Here's how the part is built. I have some questions about the finished solid (model axes, mm). Give positions to 0.01 mm unless a question says otherwise; leave off trailing zeros. Order: outer loops, then holes, each group sorted by start corner. A loop starts at its lowest first (then second) coordinate and runs counter-clockwise, first axis right, second up.
from build123d import *

# Parameters (mm, degrees)
PAD007_DEPTH    = 12
SKETCH017_R     = 4
POCKET003_DEPTH = 12.001
SKETCH042_R     = 4
HOLE009_DEPTH   = 610.001


with BuildPart() as side_left_bottom_part:
    # Sketch016 → Pad007 (new body)
    with BuildSketch(Plane.YZ):
        with BuildLine():
            ThreePointArc((-597.560459, -4876.606763), (-519.72621, -4994.682239), (-401.650734, -4916.84799))
            ThreePointArc((-401.650734, -4916.84799), (-253.112342, -4128.51152), (-130.4314, -3335.739529))
            Line((-195.221935, -3317.531256), (-130.4314, -3335.739529))
            ThreePointArc((-199.003331, -3309.149426), (-199.067813, -3314.222405), (-195.221935, -3317.531256))
            Line((-175.537372, -3260.47474), (-199.003331, -3309.149426))
            ThreePointArc((-175.537372, -3260.47474), (-175.47289, -3255.401761), (-179.318768, -3252.09291))
            Line((-244.109303, -3233.884637), (-179.318768, -3252.09291))
            ThreePointArc((-244.109303, -3233.884637), (-249.326998, -3234.856662), (-251.732171, -3239.58787))
            Line((-252.389603, -3293.61975), (-251.732171, -3239.58787))
            ThreePointArc((-260.01247, -3299.322983), (-254.794775, -3298.350957), (-252.389603, -3293.61975))
            Line((-324.803005, -3281.114709), (-260.01247, -3299.322983))
            ThreePointArc((-597.560459, -4876.606763), (-447.909647, -4081.129666), (-324.803005, -3281.114709))
        make_face()
    extrude(amount=PAD007_DEPTH)

    # Sketch017 → Pocket003 (cut, through all)
    with BuildSketch(Plane.YZ):
        with Locations((-464.310755, -4720.902056)):
            Circle(SKETCH017_R)
        with Locations((-475.70018, -4778.452535)):
            Circle(SKETCH017_R)
        with Locations((-272.113802, -3617.482184)):
            Circle(SKETCH017_R)
        with Locations((-280.914226, -3675.476508)):
            Circle(SKETCH017_R)
        with Locations((-130.873609, -2506.378514)):
            Circle(SKETCH017_R)
        with Locations((-137.037316, -2564.720482)):
            Circle(SKETCH017_R)
        with BuildLine():
            ThreePointArc((-63.5924, -1210.755644), (-69.621614, -1215.669765), (-64.707493, -1221.698978))
            Line((-64.707493, -1221.698978), (1.615745, -1228.457117))
            ThreePointArc((1.615745, -1228.457117), (7.644959, -1223.542997), (2.730838, -1217.513783))
            Line((2.730838, -1217.513783), (-63.5924, -1210.755644))
        make_face()
        with BuildLine():
            ThreePointArc((-33.541666, -94.499783), (-39.041666, -99.999783), (-33.541666, -105.499783))
            Line((-33.541666, -105.499783), (33.125001, -105.499783))
            ThreePointArc((33.125001, -105.499783), (38.625001, -99.999783), (33.125001, -94.499783))
            Line((33.125001, -94.499783), (-33.541666, -94.499783))
        make_face()
        with BuildLine():
            ThreePointArc((-165.386078, -2523.207318), (-171.913956, -2527.436597), (-167.684677, -2533.964476))
            Line((-167.684677, -2533.964476), (-102.489783, -2547.895382))
            ThreePointArc((-102.489783, -2547.895382), (-95.961904, -2543.666103), (-100.191183, -2537.138225))
            Line((-100.191183, -2537.138225), (-165.386078, -2523.207318))
        make_face()
        with BuildLine():
            ThreePointArc((-307.201152, -3631.252582), (-314.086519, -3634.870829), (-310.468272, -3641.756197))
            Line((-310.468272, -3641.756197), (-246.81, -3661.556925))
            ThreePointArc((-246.81, -3661.556925), (-239.924632, -3657.938678), (-243.542879, -3651.05331))
            Line((-243.542879, -3651.05331), (-307.201152, -3631.252582))
        make_face()
        with BuildLine():
            ThreePointArc((-498.714671, -4731.898869), (-505.894975, -4734.889394), (-502.90445, -4742.069697))
            Line((-502.90445, -4742.069697), (-441.263063, -4767.462292))
            ThreePointArc((-441.263063, -4767.462292), (-434.082759, -4764.471767), (-437.073284, -4757.291463))
            Line((-437.073284, -4757.291463), (-498.714671, -4731.898869))
        make_face()
    extrude(amount=POCKET003_DEPTH, mode=Mode.SUBTRACT)

    # Sketch042 (on Face1 of ShapeBinder002) → Hole009 (cut, through all)
    with BuildSketch(Plane.YZ.offset(610)):
        with Locations((-183.680954, -3542.695807)):
            Circle(SKETCH042_R)
        with Locations((-417.188268, -4875.410265)):
            Circle(SKETCH042_R)
    extrude(amount=-HOLE009_DEPTH, mode=Mode.SUBTRACT)


with BuildPart() as side_left_bottom_part_1:
    # Body008 placement: moved
    add(side_left_bottom_part.part.moved(Location((610, 0, 0))))


with BuildPart() as side_right_bottom_part:
    # Part__Mirroring004: instance of side_left_bottom_part
    add(side_left_bottom_part_1.part.mirror(Plane(origin=(0, 0, 0), x_dir=(0, -1, 0), z_dir=(1, 0, 0))))


solid = side_right_bottom_part.part
Q1. If we section it at C-C on y = -536: List the corners of the cut face in (x, z) for me.
Filled sheet:
outline: (-622, -4989.87) - (-610, -4989.87) - (-610, -4566.71) - (-622, -4566.71) - close
Q2. I'm going to push flat-ended pins straight in: P1, Ø5, axis at y = -464.31, z = -4720.9, coming from the +X side; P2, Ø3, axis at x = -617, z = -3646, coming from the +Y side; P3, Ø5, axis at x = -618.5, y = -224, coming from the +Z side. Where does each tip first touch, or does it pass through?
Filled sheet:
P1: passes through
P2: stops at y = -175.06
P3: stops at z = -3238.83
Q3. I need wall thicknesses on L1, parallel to Y at x = -617.25, z = -4274.5; L2, parallel to Y at x = -617, z = -3622. Which ranges of each line are inside material? Lowest first, please.
Filled sheet:
L1: y = -481.77 to -278.61
L2: y = -373.93 to -171.67
Q4. If we section it at A-A on x = -618.25: Give the number of separate pieces and of enclosed holes in the cut face, plus the area to 3 significant figures.
Filled sheet:
separate pieces: 1
enclosed holes: 8
area: 341,000 mm2
Q5. If we section it at B-B on z = -4523: List the corners of the cut face in (x, y) for me, plus the area to 3 significant figures.
Filled sheet:
outline: (-622, -527.65) - (-610, -527.65) - (-610, -324.1) - (-622, -324.1) - close
area: 2,440 mm2
